```python
from build123d import *

# Parameters (mm, degrees)
F0_R      = 12.2171028197
F1_DEPTH  = 124.206
F14_R     = 7.0299846098
F15_DEPTH = 65.786
F10_E8_W  = 77.8220303902
F10_E8_H  = 7.62
F16_DEPTH = 36.83
F11_E6_W  = 78.43691694
F11_E6_H  = 7.62
F17_DEPTH = 38.1


# Not quite as in the source:
# - the program builds the solid bodies; features that only make, move or delete a surface that nothing else refers to are left out


with BuildPart() as f1:
    # F0 (on Right) → F1 (new body)
    with BuildSketch(Plane.YZ):
        Circle(F0_R)
    extrude(amount=F1_DEPTH)

    # F14 (on Right) → F15 (join)
    with BuildSketch(Plane.YZ):
        with Locations((0, -19.1768705845)):
            Circle(F14_R)
    extrude(amount=F15_DEPTH)

    # F10_E8 (on explicit) → F16 (join)
    with BuildSketch(Plane(origin=(68.1120529771, -75.4232108593, -3.81), x_dir=(-0.5873196318, 0.8093550828, 0), z_dir=(0.8093550828, 0.5873196318, 0))):
        with Locations((38.9110151951, 3.81)):
            Rectangle(F10_E8_W, F10_E8_H)
    extrude(amount=F16_DEPTH)

    # F11_E6 (on explicit) → F17 (join)
    with BuildSketch(Plane(origin=(68.1120529771, 76.1882886291, -3.81), x_dir=(-0.5862686387, -0.8101167097, 0), z_dir=(-0.8101167097, 0.5862686387, 0))):
        with Locations((39.21845847, 3.81)):
            Rectangle(F11_E6_W, F11_E6_H)
    extrude(amount=-F17_DEPTH)


solid = f1.part
```
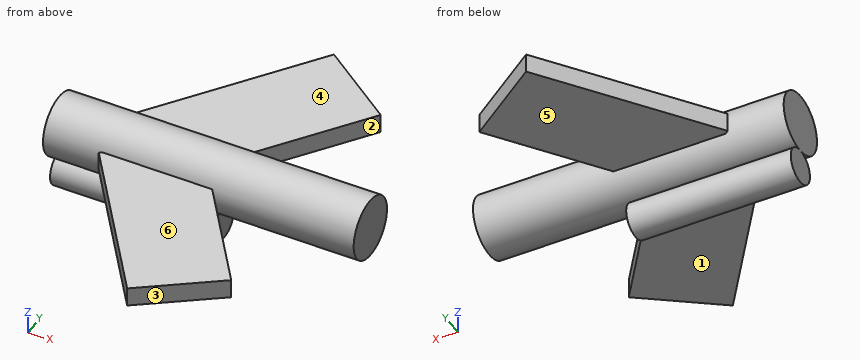
Check sheet for the modelled part. Datum: model origin and axes. Units: mm. Face numbers are marked on the shaded views. A direction names the side the tool comes from. Give positions to 0.01 mm unless a question says otherwise; leave off trailing zeros. Write each loop counter-clockwise with the first axis right and the second up, starting at its lowest first coordinate (ties: lowest second). Pieces come first, ordered by that corner, then holes.
Item 1: Cross-section at A-A (z = 0). Enter the section's corners in (x, y).
Item 2: Scan lines: L1, parallel to Z at x = 33.5, y = 23.5; L2, parallel to Y at x = 61, z = 10; L3, parallel to X at y = -60, z = 1. Record each from-to range of solid material in increasing order.
Item 3: Gauge pin test, flat ends, axial feed: pin 1 (4 mm diameter, centred on x = 35, z = -20, fed in from -Y); pin 2 (10 mm diameter, centred on x = 46.5, z = -4.5, fed in from -Y); pin 3 (7 mm diameter, centred on y = 0, z = -19.5, fed in from +X); pin 4 (12 mm diameter, centred on x = 64, z = -3.5, fed in from -Y). Record the tip position at first contact, or that the pin passes through.
Item 4: Access from +Z, -Z, +X, -X, +Y, -Y to the whole of each face (thin tool, end or side, straight path). Record for the marked faces 4, 5 and 6.
Item 5: Cross-section at C-C (y = 65). Enter the section's corners in (x, z), and give its area (3 significant figures).
Item 6: Cross-section at B-B (x = 49). Enter the section's corners in (y, z), and give its area (3 significant figures).
Item 7: Cross-section at D-D (y = -60.5). Enter the section's corners in (x, z).
Item 8: Draft check along Y on the marked faces 1, 2 and 3. Enter one of: released by +Y, released by -Y, zero draft, split by the parting line, or undercut.
Report:
1. outline: (0, -12.22) - (22.71, -12.22) - (22.41, -12.44) - (68.11, -75.42) - (97.92, -53.79) - (67.75, -12.22) - (124.21, -12.22) - (124.21, 12.22) - (68.85, 12.22) - (98.98, 53.85) - (68.11, 76.19) - (22.13, 12.65) - (22.72, 12.22) - (0, 12.22) - close
2. L1: z = -3.81 to 3.81
2. L2: y = -7.02 to 7.02
2. L3: x = 56.92 to 89.37
3. pin 1: stops at y = -7.03
3. pin 2: stops at y = -52.47
3. pin 3: stops at x = 65.79
3. pin 4: stops at y = -75.42
4. face 4: +Z, +X, -X, +Y
4. face 5: -Z, +X, -X, +Y
4. face 6: +Z, +X, -X, -Y
5. outline: (60.02, -3.81) - (83.57, -3.81) - (83.57, 3.81) - (60.02, 3.81) - close
5. area: 180 mm2
6. outline: (-49.09, -3.81) - (-11.61, -3.81) arc R12.22 ccw to (-0.79, -12.19) arc R7.03 ccw (long way) to (0.79, -12.19) arc R12.22 ccw to (11.61, -3.81) - (49.78, -3.81) - (49.78, 3.81) - (11.61, 3.81) arc R12.22 ccw to (-11.61, 3.81) - (-49.09, 3.81) - close
6. area: 1,190 mm2
7. outline: (57.28, -3.81) - (88.68, -3.81) - (88.68, 3.81) - (57.28, 3.81) - close
8. face 1: zero draft
8. face 2: undercut
8. face 3: released by -Y
